Part model, mm, in its own coordinate system. Give positions to 0.01 mm unless a question says otherwise; leave off trailing zeros. Order: outer loops, then holes, each group sorted by start corner. A loop starts at its lowest first (then second) coordinate and runs counter-clockwise, first axis right, second up. Notation, with made-up numbers: (22, -20.5) - (37, -20.5) arc R14 ccw to (37, -11.5) - close; hole circle Ø4 at (-12, 71). An arc over 180 degrees is marked (long way). One line per item, written item: value.
```python
from build123d import *

# Parameters (mm, degrees)
BOSS_EXTRUDE1_DEPTH = 50
FILLET1_R           = 10
BOSS_EXTRUDE2_DEPTH = 2.5
FILLET3_R           = 2


with BuildPart() as part:
    # Sketch1 → Boss-Extrude1 (new body)
    with BuildSketch(Plane(origin=(0, 0, 0), x_dir=(1, 0, 0), z_dir=(0, 1, 0))):
        with BuildLine():
            Line((-150, -1076.600668772), (-150, -1086.696369737))
            ThreePointArc((-150, -1086.696369737), (0, -1097), (150, -1086.696369737))
            Line((150, -1086.696369737), (150, -1076.600668772))
            ThreePointArc((150, -1076.600668772), (0, -1087), (-150, -1076.600668772))
        make_face()
    extrude(amount=BOSS_EXTRUDE1_DEPTH)

    # Fillet1
    fillet1_edges = [part.edges().sort_by_distance(p)[0] for p in [
        (150, 50, 1081.648519255),
        (150, 0, 1081.648519255),
        (-150, 0, 1081.648519255),
        (-150, 50, 1081.648519255),
    ]]
    fillet(fillet1_edges, radius=FILLET1_R)

    # Sketch3 → Boss-Extrude2 (add, symmetric)
    with BuildSketch(Plane(origin=(0, 25, 0), x_dir=(1, 0, 0), z_dir=(0, 1, 0))):
        with BuildLine():
            Line((-140, -1088.029870913), (-140.63810392, -1092.988986095))
            ThreePointArc((-140.63810392, -1092.988986095), (0, -1102), (140.63810392, -1092.988986095))
            Line((140.63810392, -1092.988986095), (140, -1088.029870913))
            ThreePointArc((140, -1088.029870913), (0, -1097), (-140, -1088.029870913))
        make_face()
    extrude(amount=BOSS_EXTRUDE2_DEPTH, both=True)

    # Fillet3
    fillet3_edges = [part.edges().sort_by_distance(p)[0] for p in [
        (-140.31905196, 22.5, 1090.509428504),
        (140.31905196, 22.5, 1090.509428504),
        (-140.31905196, 27.5, 1090.509428504),
        (140.31905196, 27.5, 1090.509428504),
    ]]
    fillet(fillet3_edges, radius=FILLET3_R)


solid = part.part
```
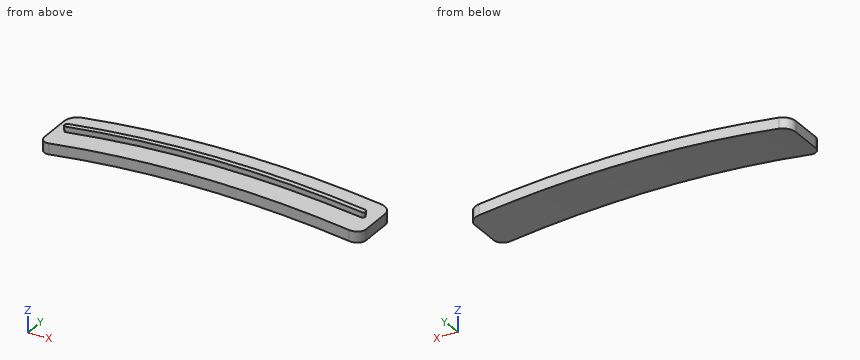
1) Cut at D-D, the plane x = -118. Give the cut face in (y, z), then the cut area to 3 significant figures.
Outcome:
outline: (0, 1080.58) - (50, 1080.58) - (50, 1090.64) - (27.5, 1090.64) - (27.5, 1095.66) - (22.5, 1095.66) - (22.5, 1090.64) - (0, 1090.64) - close
area: 528 mm^2
2) Cut at C-C, the plane y = 12.5. Give the cut face in (x, z), then the cut area to 3 significant figures.
Outcome:
outline: (-150, 1076.6) arc R1087 cw to (150, 1076.6) - (150, 1086.7) arc R1097 ccw to (-150, 1086.7) - close
area: 3,010 mm^2
3) Drill centre lines: line 1 along Y through (x, z) = (66, 1096.25); line 2 along Z through (x, y) = (-111, 28.5); line 3 along Z through (x, y) = (19, 9). Where is each one in solid material? Low to high. Write a range as from..to.
Outcome:
line 1: y = 22.5..27.5
line 2: z = 1081.32..1091.37
line 3: z = 1086.83..1096.84
4) Cut at B-B, the plane x = 51.5. Give the cut face in (y, z).
Outcome:
outline: (0, 1085.78) - (50, 1085.78) - (50, 1095.79) - (27.5, 1095.79) - (27.5, 1100.8) - (22.5, 1100.8) - (22.5, 1095.79) - (0, 1095.79) - close
